Input: part model. Units: mm. Frame: model coordinates. A direction names the side the tool comes from. Round coordinates to 2 decimals unless told otherwise and drop trailing zeros. Loops run counter-clockwise (first coordinate to the right, second up) from the corner with the lowest first, then second, coordinate; pieces in that order, holes last. Notation, with made-up numbers: (22, 2) -> (77, 2) arc R24 ccw to (77, 27) -> close; hole circle Ø9 at (12, 8). An arc over 180 degrees is marked (long way). Answer as a JSON object with one key per item and string values. Group by question number.
Item 1: Section query B-B on x = -15. Return loops of the section in (y, z).
Item 2: Section query A-A on y = 10. Return loops of the section in (x, z).
Item 3: Set-up query: faces 4 (the flat face through (-55, 7, 1)), 5 (the flat face through (-31, 32, 2)), 6 (the flat face through (51, 30.5, 1)), 7 (the flat face through (-13, -30.5, 1)), 8 (the flat face through (-38, -30.5, 1)). Return all of +Z, -Z, +X, -X, +Y, -Y with unobstructed straight access to the full face (end or side cutting, diameter ignored); none if empty.
Item 4: Pin query (flat end, axial travel): pin 1 (1.5 mm diameter, centred on x = 3.5, y = 19.5, fed in from -Z); pin 2 (1.5 mm diameter, centred on y = 0.5, z = 0.5, fed in from +X); pin 3 (1.5 mm diameter, centred on x = 40, z = 1.5, fed in from +Y); pin 4 (1.5 mm diameter, centred on y = -20, z = 1.5, fed in from +X). Return the tip coordinate at first contact, or that it passes through.
Item 5: Material intervals for line 1 (X direction, y = -28, z = 0.95); line 2 (X direction, y = 30, z = 1); line 3 (X direction, y = -12, z = 0.85), sorted ascending. Write a range as [from, to].
Item 6: Draft query along Y for faces 1 (the flat face through (38, 30.5, 1)), 2 (the flat face through (38, -30.5, 1)), 3 (the cylindrical face through (35.6, -0.1, 1.5)). Return one class per face: released by +Y, released by -Y, zero draft, split by the parting line, or undercut.
from build123d import *

# Parameters (mm, degrees)
BOSS_EXTRUDE1_DEPTH = 3
CUT_EXTRUDE1_DEPTH  = 3
CUT_EXTRUDE3_DEPTH  = 3
FILLET2_R           = 1
CUT_EXTRUDE4_DEPTH  = 10
FILLET3_R           = 3
SKETCH5_W           = 3
SKETCH5_H           = 7
SKETCH5_W_2         = 7
SKETCH5_H_2         = 3
BOSS_EXTRUDE2_DEPTH = 3


with BuildPart() as part:
    # Sketch1 → Boss-Extrude1 (new body)
    with BuildSketch(Plane.XY):
        with BuildLine():
            Line((55, 30.5), (-55, 30.5))
            Line((-55, 30.5), (-55, 1.5))
            Line((-55, 1.5), (-47, 1.5))
            Line((-47, 1.5), (-47, 2))
            Line((-47, 2), (-47, 3))
            Line((-47, 3), (-46, 3))
            Line((-46, 3), (-45.6, 3))
            Line((-45.6, 3), (-44.6, 3))
            Line((-44.6, 3), (-44.6, 2))
            Line((-44.6, 2), (-44.6, 1.5))
            ThreePointArc((-44.6, 1.5), (-43.1, 0), (-44.6, -1.5))
            Line((-44.6, -1.5), (-44.6, -2))
            Line((-44.6, -2), (-44.6, -3))
            Line((-44.6, -3), (-45.6, -3))
            Line((-45.6, -3), (-46, -3))
            Line((-46, -3), (-47, -3))
            Line((-47, -3), (-47, -2))
            Line((-47, -2), (-47, -1.5))
            Line((-47, -1.5), (-55, -1.5))
            Line((-55, -1.5), (-55, -30.5))
            Line((-55, -30.5), (55, -30.5))
            Line((55, -30.5), (55, -1.5))
            Line((55, -1.5), (47, -1.5))
            Line((47, -1.5), (47, -2))
            Line((47, -2), (47, -3))
            Line((47, -3), (46, -3))
            Line((46, -3), (45.6, -3))
            Line((45.6, -3), (44.6, -3))
            Line((44.6, -3), (44.6, -2))
            Line((44.6, -2), (44.6, -1.5))
            ThreePointArc((44.6, -1.5), (43.1, 0), (44.6, 1.5))
            Line((44.6, 1.5), (44.6, 2))
            Line((44.6, 2), (44.6, 3))
            Line((44.6, 3), (45.6, 3))
            Line((45.6, 3), (46, 3))
            Line((46, 3), (47, 3))
            Line((47, 3), (47, 2))
            Line((47, 2), (47, 1.5))
            Line((47, 1.5), (55, 1.5))
            Line((55, 1.5), (55, 30.5))
        make_face()
        with BuildLine():
            ThreePointArc((-46, -3), (-46.707106781, -2.707106781), (-47, -2))
            Line((-47, -2), (-47, -3))
            Line((-47, -3), (-46, -3))
        make_face()
        with BuildLine():
            ThreePointArc((-44.6, -2), (-44.892893219, -2.707106781), (-45.6, -3))
            Line((-45.6, -3), (-44.6, -3))
            Line((-44.6, -3), (-44.6, -2))
        make_face()
        with BuildLine():
            Line((-44.6, 3), (-45.6, 3))
            ThreePointArc((-45.6, 3), (-44.892893219, 2.707106781), (-44.6, 2))
            Line((-44.6, 2), (-44.6, 3))
        make_face()
        with BuildLine():
            Line((-47, 3), (-47, 2))
            ThreePointArc((-47, 2), (-46.707106781, 2.707106781), (-46, 3))
            Line((-46, 3), (-47, 3))
        make_face()
        with BuildLine():
            Line((44.6, -3), (45.6, -3))
            ThreePointArc((45.6, -3), (44.892893219, -2.707106781), (44.6, -2))
            Line((44.6, -2), (44.6, -3))
        make_face()
        with BuildLine():
            Line((47, -3), (47, -2))
            ThreePointArc((47, -2), (46.707106781, -2.707106781), (46, -3))
            Line((46, -3), (47, -3))
        make_face()
        with BuildLine():
            ThreePointArc((46, 3), (46.707106781, 2.707106781), (47, 2))
            Line((47, 2), (47, 3))
            Line((47, 3), (46, 3))
        make_face()
        with BuildLine():
            ThreePointArc((44.6, 2), (44.892893219, 2.707106781), (45.6, 3))
            Line((45.6, 3), (44.6, 3))
            Line((44.6, 3), (44.6, 2))
        make_face()
    extrude(amount=BOSS_EXTRUDE1_DEPTH)

    # Sketch2 → Cut-Extrude1 (cut)
    with BuildSketch(Plane.XY.offset(3)):
        with BuildLine():
            Line((45.136675042, 30.5), (44.6, 30.5))
            Line((44.6, 30.5), (44.6, 29.5))
            ThreePointArc((44.6, 29.5), (45.8, 28.3), (47, 29.5))
            Line((47, 29.5), (47, 30.5))
            Line((47, 30.5), (46.463324958, 30.5))
            Line((46.463324958, 30.5), (45.136675042, 30.5))
        make_face()
        with BuildLine():
            Line((44.6, -29.5), (44.6, -30.5))
            Line((44.6, -30.5), (45.136675042, -30.5))
            Line((45.136675042, -30.5), (46.463324958, -30.5))
            Line((46.463324958, -30.5), (47, -30.5))
            Line((47, -30.5), (47, -29.5))
            ThreePointArc((47, -29.5), (45.8, -28.3), (44.6, -29.5))
        make_face()
        with BuildLine():
            ThreePointArc((-44.6, -29.5), (-45.8, -28.3), (-47, -29.5))
            Line((-47, -29.5), (-47, -30.5))
            Line((-47, -30.5), (-46.463324958, -30.5))
            Line((-46.463324958, -30.5), (-45.136675042, -30.5))
            Line((-45.136675042, -30.5), (-44.6, -30.5))
            Line((-44.6, -30.5), (-44.6, -29.5))
        make_face()
        with BuildLine():
            Line((-47, 30.5), (-47, 29.5))
            ThreePointArc((-47, 29.5), (-45.8, 28.3), (-44.6, 29.5))
            Line((-44.6, 29.5), (-44.6, 30.5))
            Line((-44.6, 30.5), (-45.136675042, 30.5))
            Line((-45.136675042, 30.5), (-46.463324958, 30.5))
            Line((-46.463324958, 30.5), (-47, 30.5))
        make_face()
    extrude(amount=-CUT_EXTRUDE1_DEPTH, mode=Mode.SUBTRACT)

    # Sketch3 → Cut-Extrude3 (cut)
    with BuildSketch(Plane.XY.offset(3)):
        with BuildLine():
            ThreePointArc((1.5, -20.1), (0, -18.6), (-1.5, -20.1))
            Line((-1.5, -20.1), (-3, -20.1))
            Line((-3, -20.1), (-3, -22.5))
            Line((-3, -22.5), (-1.5, -22.5))
            Line((-1.5, -22.5), (-1.5, -30.5))
            Line((-1.5, -30.5), (0, -30.5))
            Line((0, -30.5), (1.5, -30.5))
            Line((1.5, -30.5), (1.5, -22.5))
            Line((1.5, -22.5), (3, -22.5))
            Line((3, -22.5), (3, -20.1))
            Line((3, -20.1), (1.5, -20.1))
        make_face()
    extrude(amount=-CUT_EXTRUDE3_DEPTH, mode=Mode.SUBTRACT)

    # Fillet2
    fillet2_edges = [part.edges().sort_by_distance(p)[0] for p in [
        (3, -20.1, 1.5),
        (3, -22.5, 1.5),
        (-3, -22.5, 1.5),
        (-3, -20.1, 1.5),
    ]]
    fillet(fillet2_edges, radius=FILLET2_R)

    # Sketch4 → Cut-Extrude4 (cut)
    with BuildSketch(Plane.XY.offset(3)):
        with BuildLine():
            Line((40, 20.5), (-40, 20.5))
            Line((-40, 20.5), (-40, 6.829348432))
            ThreePointArc((-40, 6.829348432), (-36.795239894, 4.062019202), (-35.6, 0))
            ThreePointArc((-35.6, 0), (-36.795239894, -4.062019202), (-40, -6.829348432))
            Line((-40, -6.829348432), (-40, -15.5))
            Line((-40, -15.5), (-6.829348432, -15.5))
            ThreePointArc((-6.829348432, -15.5), (0, -11.1), (6.829348432, -15.5))
            Line((6.829348432, -15.5), (40, -15.5))
            Line((40, -15.5), (40, -6.829348432))
            ThreePointArc((40, -6.829348432), (35.6, 0), (40, 6.829348432))
            Line((40, 6.829348432), (40, 20.5))
        make_face()
    extrude(amount=-CUT_EXTRUDE4_DEPTH, mode=Mode.SUBTRACT)

    # Fillet3
    fillet3_edges = [part.edges().sort_by_distance(p)[0] for p in [
        (40, 6.829348432, 1.5),
        (40, -6.829348432, 1.5),
        (40, -15.5, 1.5),
        (6.829348432, -15.5, 1.5),
        (-6.829348432, -15.5, 1.5),
        (-40, -15.5, 1.5),
        (-40, -6.829348432, 1.5),
        (-40, 6.829348432, 1.5),
        (-40, 20.5, 1.5),
        (40, 20.5, 1.5),
    ]]
    fillet(fillet3_edges, radius=FILLET3_R)

    # Sketch5 → Boss-Extrude2 (add)
    with BuildSketch(Plane.XY.offset(3)):
        with Locations((-56.5, 15.25)):
            Rectangle(SKETCH5_W, SKETCH5_H)
        with Locations((-56.5, -15.25)):
            Rectangle(SKETCH5_W, SKETCH5_H)
        with Locations((56.5, -15.25)):
            Rectangle(SKETCH5_W, SKETCH5_H)
        with Locations((56.5, 15.25)):
            Rectangle(SKETCH5_W, SKETCH5_H)
        with Locations((27.5, -32)):
            Rectangle(SKETCH5_W_2, SKETCH5_H_2)
        with Locations((-27.5, -32)):
            Rectangle(SKETCH5_W_2, SKETCH5_H_2)
        with Locations((-27.5, 32)):
            Rectangle(SKETCH5_W_2, SKETCH5_H_2)
        with Locations((27.5, 32)):
            Rectangle(SKETCH5_W_2, SKETCH5_H_2)
    extrude(amount=-BOSS_EXTRUDE2_DEPTH)


solid = part.part
Solved:
{
 "1": {"outline": "(-30.5, 0) -> (-15.5, 0) -> (-15.5, 3) -> (-30.5, 3) -> close; (20.5, 0) -> (30.5, 0) -> (30.5, 3) -> (20.5, 3) -> close"},
 "2": {"outline": "(-55, 0) -> (-40, 0) -> (-40, 3) -> (-55, 3) -> close; (40, 0) -> (55, 0) -> (55, 3) -> (40, 3) -> close"},
 "3": {"face 4": "+Z, -Z, -X", "face 5": "+Z, -Z, -X, +Y", "face 6": "+Z, -Z, +X, +Y", "face 7": "+Z, -Z, -Y", "face 8": "+Z, -Z, -X, -Y"},
 "4": {"pin 1": "through", "pin 2": "x = 43.77", "pin 3": "y = 30.5", "pin 4": "x = 55"},
 "5": {"line 1": "[-55, -1.5], [1.5, 55]", "line 2": "[-55, -47], [-44.6, 44.6], [47, 55]", "line 3": "[-58, -40], [-3.56, 3.56], [40, 58]"},
 "6": {"face 1": "released by +Y", "face 2": "released by -Y", "face 3": "undercut"}
}
